Autodesk Inventor part; units mm, degrees
ref_plane "YZ Plane" through (0, 0, 0) normal (1, 0, 0) x (0, 1, 0)
ref_plane "XZ Plane" through (0, 0, 0) normal (0, 1, 0) x (-1, 0, 0)
ref_plane "XY Plane" through (0, 0, 0) normal (0, 0, 1) x (1, 0, 0)
sketch "Sketch1" plane through (0, 0, 0) normal (0, 0, 1) x (1, 0, 0)
  line L0 (18.5, -17.5) -> (-18.5, -17.5)
  line L1 (-18.5, -17.5) -> (-18.5, 17.5)
  line L2 (-18.5, 17.5) -> (18.5, 17.5)
  line L3 (18.5, 17.5) -> (18.5, -17.5)
  line L4 (18.5, -17.5) -> (-18.5, 17.5) construction
  line L5 (-18.5, -17.5) -> (18.5, 17.5) construction
  line L6 (0, 14.9312) -> (16, -12.7816) construction
  line L7 (16, -12.7816) -> (-16, -12.7816) construction
  line L8 (-16, -12.7816) -> (0, 14.9312) construction
  line L9 (-9.3116, -12.7816) -> (0.017, 3.3758) construction
  line L10 (0.017, 3.3758) -> (9.3455, -12.7816) construction
  line L11 (9.3455, -12.7816) -> (-9.3116, -12.7816) construction
  circle A0 centre (0, 14.9312) radius 1.4
  circle A1 centre (16, -12.7816) radius 1.4
  circle A2 centre (9.3455, -12.7816) radius 1.4
  circle A3 centre (0.017, 3.3758) radius 1.4
  circle A4 centre (-9.3116, -12.7816) radius 1.4
  line L12 (-4.6002, 17.5) -> (-18.5, -6.5752)
  line L13 (18.5, -6.5752) -> (4.6002, 17.5)
  point P0 (0, 0)
  point P1 (0, -3.544)
  point P2 (0.017, -7.3958)
  dimension "d0" = 37
  dimension "d1" = 35
  dimension "d3" = 32
  dimension "d4" = 0
  dimension "d5" = 2.8
  dimension "d6" = 2.8
  dimension "d7" = 2.8
  dimension "d8" = 2.8
  dimension "d9" = 2.8
extrude "Extrusion1" add sketch "Sketch1" along normal blind 10 contours L0 L1 L12 L2 L13 L3
properties part number "cellSTORM_chip_Adapter_screws"
Source: CAD feature listing. Evaluate the final solid. Frame: model axes, mm. Coordinates: 2 decimals unless noted, no trailing zeros. Loops run counter-clockwise (first coordinate to the right, second up) from the corner with the lowest first, then second, coordinate; pieces in that order, holes last. Notation, with made-up numbers: (0, 7.25) -> (39, 7.25) arc R28 ccw to (39, 27.25) -> close; hole circle Ø7 at (81.5, -23). An arc over 180 degrees is marked (long way). One line per item, written item: value. Start each with the question number.
Q1. Section query C-C, the plane x = 16. Return the cut outline in (y, z).
Q2. Section query B-B, the plane z = 7.5. Return the cut outline in (x, y).
Q3. Contact query for flat-ended pins moving along their axis: P1, Ø5, axis at y = 1.5, z = 8.5, coming from the +X side; P2, Ø4, axis at x = 10, z = 7, coming from the +Y side. Output: stop coordinate, or through.
Q4. Section query A-A, the plane x = 0. Return the cut outline in (y, z).
Q5. Mould query, pull axis X, two halves, no side actions, for faces 1 (the face through (-10.4, -11.9, 4.9)), 2 (the face through (0, 17.5, 5)), 3 (the face through (18.5, -12, 5)), 4 (the face through (-0.29, 4.74, 4.93)). Classes: pulls with the +X half, pulls with the -X half, needs draft (parallel to the pull), parting line crosses it, or undercut.
Q6. Section query D-D, the plane y = 9. Return the cut outline in (x, z).
Q7. Line query: line 1 along Y through (x, z) = (0, 3.5); line 2 along X through (y, z) = (-13.5, 8.5); line 3 along X through (y, z) = (2.5, 5). Output: solid intervals per line, ascending.
Results:
1. outline: (-17.5, 0) -> (-14.18, 0) -> (-14.18, 10) -> (-17.5, 10) -> close; (-11.38, 0) -> (-2.25, 0) -> (-2.25, 10) -> (-11.38, 10) -> close
2. outline: (-18.5, -17.5) -> (18.5, -17.5) -> (18.5, -6.58) -> (4.6, 17.5) -> (-4.6, 17.5) -> (-18.5, -6.58) -> close; hole circle Ø2.8 at (-9.31, -12.78); hole circle Ø2.8 at (0, 14.93); hole circle Ø2.8 at (0.02, 3.38); hole circle Ø2.8 at (9.35, -12.78); hole circle Ø2.8 at (16, -12.78)
3. P1: x = 15.28
3. P2: y = 11.61
4. outline: (-17.5, 0) -> (1.98, 0) -> (1.98, 10) -> (-17.5, 10) -> close; (4.78, 0) -> (13.53, 0) -> (13.53, 10) -> (4.78, 10) -> close; (16.33, 0) -> (17.5, 0) -> (17.5, 10) -> (16.33, 10) -> close
5. face 1: undercut
5. face 2: needs draft
5. face 3: pulls with the +X half
5. face 4: undercut
6. outline: (-9.51, 0) -> (9.51, 0) -> (9.51, 10) -> (-9.51, 10) -> close
7. line 1: -17.5 to 1.98, 4.78 to 13.53, 16.33 to 17.5
7. line 2: -18.5 to -10.51, -8.11 to 8.14, 10.55 to 14.8, 17.2 to 18.5
7. line 3: -13.26 to -1.08, 1.11 to 13.26
